Work out the finished part from the listing and answer in its coordinate system (mm). A direction names the side the tool comes from. Coordinates: 2 decimals unless noted, no trailing zeros. Loops run counter-clockwise (first coordinate to the right, second up) from the corner with the lowest first, then second, coordinate; pieces in that order, holes last. Notation, with made-up numbers: (39, 23) -> (60, 23) arc R16 cw to (60, 52) -> close; hole circle Ø11 at (74.25, 49.25). An arc over 180 degrees is marked (long way). Use a Markdown table: item, result.
from build123d import *

# Parameters (mm, degrees)
F0_R     = 5.5
F1_DEPTH = 7.8
F2_R     = 4
F2_R_2   = 2.5
F2_R_3   = 1.05
F3_DEPTH = 6
F6_DEPTH = 2
F7_W     = 0.456778
F7_H     = 2.030816
F7_W_2   = 2.131754
F7_H_2   = 0.43523
F7_H_3   = 0.434156
F8_DEPTH = 8.5


with BuildPart() as f1:
    # F0 (on Front) → F1 (new body)
    with BuildSketch(Plane.XZ):
        Circle(F0_R)
    extrude(amount=-F1_DEPTH)

    # F2 (on Front) → F3 (join)
    with BuildSketch(Plane.XZ):
        Circle(F2_R)
        Circle(F2_R_2, mode=Mode.SUBTRACT)
        Circle(F2_R_3)
    extrude(amount=F3_DEPTH)

    # F5 (on offset) → F6 (join)
    with BuildSketch(Plane.XZ.offset(4)):
        Polygon((5, -2.886751), (5, 2.886751), (0, 5.773503), (-5, 2.886751), (-5, -2.886751), (0, -5.773503), align=None)
    extrude(amount=-F6_DEPTH)

    # F7 (on face) → F8 (join)
    with BuildSketch(Plane(origin=(0, 7.8, 0), x_dir=(-1, 0, 0), z_dir=(0, 1, 0))):
        with Locations((-4, 0)):
            Rectangle(F7_W, F7_H)
        with Locations((0, 4)):
            Rectangle(F7_W_2, F7_H_2)
        with Locations((0, -4)):
            Rectangle(F7_W_2, F7_H_3)
    extrude(amount=F8_DEPTH)


solid = f1.part
Q1. Section D-D on x = 2.75 is taken. Determine the outline of the cut face in (y, z).
Solved:
| item | result |
|---|---|
| outline | (-6, -2.9) -> (-4, -2.9) -> (-4, -4.19) -> (-2, -4.19) -> (-2, -2.9) -> (0, -2.9) -> (0, -4.76) -> (7.8, -4.76) -> (7.8, 4.76) -> (0, 4.76) -> (0, 2.9) -> (-2, 2.9) -> (-2, 4.19) -> (-4, 4.19) -> (-4, 2.9) -> (-6, 2.9) -> close |
Q2. Section A-A on y = 12.75 is taken. Determine the outline of the cut face in (x, z).
Solved:
| item | result |
|---|---|
| outline | (-1.07, -4.22) -> (1.07, -4.22) -> (1.07, -3.78) -> (-1.07, -3.78) -> close; (-1.07, 3.78) -> (1.07, 3.78) -> (1.07, 4.22) -> (-1.07, 4.22) -> close; (3.77, -1.02) -> (4.23, -1.02) -> (4.23, 1.02) -> (3.77, 1.02) -> close |
Q3. Consider line 1 (Z direction, x = 0, y = -5.45); line 2 (Y direction, x = 2.25, z = 0.25). Determine where each line is inside the solid, lowest interval first. Write a range as [from, to].
Solved:
| item | result |
|---|---|
| line 1 | [-4, -2.5], [-1.05, 1.05], [2.5, 4] |
| line 2 | [-4, -2], [0, 7.8] |
Q4. Determine the mould class of faces 1 (the flat face through (0, -6, 0)), 2 (the cylindrical face through (1, -4.99, 0.32)), 3 (the flat face through (5, -3, 0)) for opening direction X: pulls with the +X half, pulls with the -X half, needs draft (parallel to the pull), parting line crosses it, or undercut.
Solved:
| item | result |
|---|---|
| face 1 | needs draft |
| face 2 | undercut |
| face 3 | pulls with the +X half |
Q5. Section C-C on y = -0.25 is taken. Determine the outline of the cut face in (x, z).
Solved:
| item | result |
|---|---|
| outline | circle Ø8 at (0, 0); circle Ø2.1 at (0, 0); hole circle Ø5 at (0, 0) |
Q6. Given pin 1 Ø5.5 at (x, z) = (0.5, -0.5) entering from +Y; pin 2 Ø4 at (x, z) = (-0.5, 1) entering from -Y; pin 3 Ø6 at (x, y) = (3, 3) entering from +Z; pin 4 Ø4 at (y, z) = (0, -2.5) entering from -X, each flat-ended and moving along its own axis, determine where each tip first touches the part or whether it passes through.
Solved:
| item | result |
|---|---|
| pin 1 | y = 7.8 |
| pin 2 | y = -6 |
| pin 3 | z = 5.5 |
| pin 4 | x = -5.48 |
Q7. For faces 4 (the flat face through (4.228, 12, 0)), 5 (the flat face through (-2.535, -3.014, -4.31)), 6 (the flat face through (2.535, -3.014, 4.31)), 7 (the flat face through (0, 12, 3.782)), 8 (the cylindrical face through (1, -0.99, 0.32)), determine the directions among +Z, -Z, +X, -X, +Y, -Y from which every point of the face is accessible in a straight line to the end or side of a thin tool.
Solved:
| item | result |
|---|---|
| face 4 | +Z, -Z, +X, +Y |
| face 5 | -Z, -X, -Y |
| face 6 | +Z, +X, -Y |
| face 7 | +X, -X, +Y |
| face 8 | none |
Q8. Section B-B on z = 2.25 is taken. Determine the outline of the cut face in (x, y), and give its area (3 significant figures).
Solved:
| item | result |
|---|---|
| outline | (-5.02, 0) -> (-3.31, 0) -> (-3.31, -2) -> (-5, -2) -> (-5, -4) -> (-3.31, -4) -> (-3.31, -6) -> (-1.09, -6) -> (-1.09, -4) -> (1.09, -4) -> (1.09, -6) -> (3.31, -6) -> (3.31, -4) -> (5, -4) -> (5, -2) -> (3.31, -2) -> (3.31, 0) -> (5.02, 0) -> (5.02, 7.8) -> (-5.02, 7.8) -> close; hole (-1.09, -2) -> (1.09, -2) -> (1.09, 0) -> (-1.09, 0) -> close |
| area | 116 mm² |
